Work out the finished part from the listing and answer in its coordinate system (mm). A direction names the side the tool comes from. Give positions to 0.01 mm unless a question says otherwise; leave off trailing zeros. Order: outer loops, then holes, each group sorted by start corner. A loop starts at its lowest first (then second) coordinate and runs counter-clockwise, first axis right, second up. Notation, with made-up numbers: M 3.5,-0.5 L 7.5,-0.5 A10 cw 7.5,4.5 Z; hole C 24.25,-4.75 d8. An arc over 180 degrees is marked long. One line per item, written item: value.
Autodesk Inventor part; units mm, degrees
ref_plane "YZ Plane" through (0, 0, 0) normal (1, 0, 0) x (0, 1, 0)
ref_plane "XZ Plane" through (0, 0, 0) normal (0, 1, 0) x (-1, 0, 0)
ref_plane "XY Plane" through (0, 0, 0) normal (0, 0, 1) x (1, 0, 0)
sketch "스케치1" plane through (0, 0, 0) normal (0, 1, 0) x (-1, 0, 0)
  line L0 (22.5, -14) -> (-22.5, -14)
  line L1 (-22.5, -14) -> (-22.5, 14)
  line L2 (-22.5, 14) -> (22.5, 14)
  line L3 (22.5, 14) -> (22.5, -14)
  point P0 (0, 0)
  dimension "d0" = 28
  dimension "d1" = 45
  dimension "d2" = 14
  dimension "d3" = 22.5
extrude "돌출1" add sketch "스케치1" along normal blind 5
sketch "스케치2" plane through (0, 5, 0) normal (0, 1, 0) x (1, 0, 0)
  circle A0 centre (18.5, 0) radius 5
  line L0 (18.5, 5) -> (22.5, 5)
  line L1 (22.5, 5) -> (22.5, -5)
  line L2 (22.5, -5) -> (18.5, -5)
  line L3 (18.5, -5) -> (18.5, 5)
  line L4 (22.5, -14) -> (22.5, 14)
  point P0 (0, 0)
  dimension "d6" = 10
  dimension "d7" = 0
  dimension "d8" = 10
  dimension "d9" = 5
  dimension "d10" = 4
  dimension "d11" = 0
extrude "돌출2" cut sketch "스케치2" against normal blind 100
sketch "스케치3" plane through (0, 5, 0) normal (0, 1, 0) x (1, 0, 0)
  circle A0 centre (19.5, 11) radius 1.25
  line L0 (22.5, 5) -> (22.5, 14)
  line L1 (22.5, 14) -> (-22.5, 14)
  line L2 (0, 0) -> (4.9885, 0)
  circle A1 centre (19.5, -11) radius 1.25
  circle A2 centre (8.5, 0) radius 1.25
  line L3 (-22.5, -14) -> (22.5, -14)
  circle A3 centre (11.722, -7.778) radius 1.25
  line L4 (22.5, -14) -> (22.5, -5)
  circle A4 centre (11.722, 7.778) radius 1.25
  dimension "d14" = 2.5
  dimension "d15" = 3
  dimension "d16" = 3
  dimension "d17" = 14
  dimension "d18" = 2.5
  dimension "d19" = 14
  dimension "d20" = 10.778
  dimension "d21" = 6.222
  dimension "d22" = 2.5
extrude "돌출3" cut sketch "스케치3" against normal blind 5
fillet "모깎기1" radius 2 4 edges at (22.5, 2.5, -14) (22.5, 2.5, 14) (22.5, 2.5, -5) (22.5, 2.5, 5)
sketch "스케치4" plane through (0, 0, 0) normal (0, -1, 0) x (1, 0, 0)
  line L0 (-22.5, -14) -> (20.5, -14)
  line L1 (20.5, 14) -> (-22.5, 14)
  line L2 (-22.5, -14) -> (-17.5, -14)
  line L3 (-17.5, -14) -> (-17.5, 14)
  line L4 (-17.5, 14) -> (-22.5, 14)
  line L5 (-22.5, 14) -> (-22.5, -14)
  point P0 (0, 0)
  dimension "d26" = 5
extrude "돌출4" add sketch "스케치4" along normal blind 52
fillet "모깎기2" radius 2 1 edges at (-22.5, 5, 0)
sketch "스케치5" plane through (-17.5, 0, 14) normal (1, 0, 0) x (0, 0, -1)
  point P0 (14, 0)
sketch "스케치6" plane through (-17.5, 0, 14) normal (1, 0, 0) x (0, 0, -1)
  line L0 (28, 0) -> (28, -52)
  line L1 (0, 0) -> (0, -52)
  line L2 (28, -52) -> (0, -52)
  line L3 (0, -52) -> (0, -47)
  line L4 (0, -47) -> (28, -47)
  line L5 (28, -47) -> (28, -52)
  point P0 (14, 0)
  dimension "d30" = 5
extrude "돌출5" add sketch "스케치6" along normal blind 40
sketch "스케치7" plane through (0, 0, 0) normal (0, -1, 0) x (1, 0, 0)
  circle A0 centre (19.5, -11) radius 1.25
  circle A1 centre (19.5, -11) radius 1.25
  circle A2 centre (11.722, -7.778) radius 1.25
  circle A3 centre (11.722, -7.778) radius 1.25
  circle A4 centre (8.5, 0) radius 1.25
  circle A5 centre (8.5, 0) radius 1.25
  circle A6 centre (11.722, 7.778) radius 1.25
  circle A7 centre (11.722, 7.778) radius 1.25
  circle A8 centre (19.5, 11) radius 1.25
  circle A9 centre (19.5, 11) radius 1.25
  arc A10 (18.5, 5) -> (18.5, -5) centre (18.5, 0) ccw
  circle A11 centre (18.5, 0) radius 5
  line L0 (18.5, -5) -> (29.1098, -5)
  line L1 (29.1098, -5) -> (29.1098, 5)
  line L2 (29.1098, 5) -> (18.5, 5)
  line L3 (18.5, 5) -> (18.5, -5)
  point P0 (0, 0)
extrude "돌출6" cut sketch "스케치7" along normal blind 200
fillet "모깎기4" radius 2 2 edges at (22.5, -49.5, 14) (22.5, -49.5, -14)
fillet "모깎기5" radius 2 1 edges at (-22.5, -52, 0)
sketch "스케치10" plane through (20.5, 0, 14) normal (0, 0, 1) x (1, 0, 0)
  circle A0 centre (-41, -12.5) radius 1.5
  circle A1 centre (-41, -34.5) radius 1.5
  line L0 (-32.0554, -23.5) -> (-2.5003, -23.5)
  line L1 (-43, 3) -> (-43, -50)
  point P0 (-20.5, 0)
  dimension "d54" = 3
  dimension "d55" = 3
  dimension "d56" = 22
  dimension "d57" = 23.5
  dimension "d58" = 11
  dimension "d59" = 2
  dimension "d60" = 2
extrude "돌출9" cut sketch "스케치10" against normal blind 80
sketch "스케치11" plane through (-17.5, 0, 14) normal (1, 0, 0) x (0, 0, -1)
  line L0 (5, -42) -> (23, -42)
  line L1 (23, -42) -> (23, -5)
  line L2 (23, -5) -> (5, -5)
  line L3 (5, -5) -> (5, -42)
  line L4 (0, 0) -> (0, -47)
  line L5 (28, 0) -> (28, -47)
  line L6 (19, 0) -> (9, 0)
  line L7 (9, -47) -> (19, -47)
  line L8 (11, -42) -> (17, -42)
  line L9 (17, -42) -> (17, -5)
  line L10 (17, -5) -> (11, -5)
  line L11 (11, -5) -> (11, -42)
  point P0 (14, 0)
  dimension "d63" = 5
  dimension "d64" = 5
  dimension "d65" = 5
  dimension "d66" = 5
  dimension "d67" = 6
  dimension "d68" = 6
extrude "돌출10" cut sketch "스케치11" against normal blind 80 contours L3 L2 L11 L0 | L9 L2 L1 L0
sketch "스케치12" plane through (-17.5, -42, 3) normal (0, 0, 1) x (1, 0, 0)
  circle A0 centre (-3, 7.5) radius 1.5
  circle A1 centre (-3, 7.5) radius 1.5
  circle A2 centre (-3, 29.5) radius 1.5
  circle A3 centre (-3, 29.5) radius 1.5
  point P0 (17.5, 42)
extrude "돌출11" add sketch "스케치12" against normal blind 6
properties part number "elbow_gear"
(1) Section D-D, the plane z = 0 is taken. Give the vertices of the cut face in (x, y), then the cut area to 3 significant figures.
Findings:
outline: M -22.5,-50 A2 ccw -20.5,-52 L 7.25,-52 L 7.25,-47 L -17.5,-47 L -17.5,0 L 7.25,0 L 7.25,5 L -20.5,5 A2 ccw -22.5,3 Z; M 9.75,-52 L 13.5,-52 L 13.5,-47 L 9.75,-47 Z; M 9.75,0 L 13.5,0 L 13.5,5 L 9.75,5 Z
area: 568 mm^2
(2) Find the intervals of material crossed by probe 1 along Z at (x, y) = (19.5, -50.55); probe 2 along Z at (x, y) = (-19, -18.5); probe 3 along Y at (x, z) = (-10, -10), in increasing order. Write a range as from..to.
Findings:
probe 1: z = -14..-12.25, -9.75..-5, 5..9.75, 12.25..14
probe 2: z = -14..-9, -3..3, 9..14
probe 3: y = -52..-47, 0..5
(3) Determine the mould class of faces 1 (the flat face through (22.5, 2, 9)), 2 (the cylindrical face through (20.69, -49.46, 10.62)), 3 (the flat face through (-19, -23, 14)), 4 (the cylindrical face through (12.299, 2.535, 8.887)) for opening direction Z: pulls with the +Z half, pulls with the -Z half, needs draft (parallel to the pull), parting line crosses it, or undercut.
Findings:
face 1: needs draft
face 2: undercut
face 3: pulls with the +Z half
face 4: undercut
(4) Section C-C, the plane y = -23.5 is taken. Give the vertices of the cut face in (x, z).
Findings:
outline: M -22.5,-14 L -17.5,-14 L -17.5,-9 L -22.5,-9 Z; M -22.5,-3 L -17.5,-3 L -17.5,3 L -22.5,3 Z; M -22.5,9 L -17.5,9 L -17.5,14 L -22.5,14 Z
(5) Section A-A, the plane z = 11 is taken. Give the vertices of the cut face in (x, y), then the cut area to 3 significant figures.
Findings:
outline: M -22.5,-50 A2 ccw -20.5,-52 L 18.25,-52 L 18.25,-47 L -17.5,-47 L -17.5,0 L 18.25,0 L 18.25,5 L -20.5,5 A2 ccw -22.5,3 Z; M 20.75,-52 L 22.5,-52 L 22.5,-47 L 20.75,-47 Z; M 20.75,0 L 22.5,0 L 22.5,5 L 20.75,5 Z; hole C -20.5,-34.5 d3; hole C -20.5,-12.5 d3
area: 644 mm^2
(6) Section B-B, the plane x = -15.5 is taken. Give the vertices of the cut face in (y, z).
Findings:
outline: M -52,-14 L -47,-14 L -47,14 L -52,14 Z; M 0,-14 L 5,-14 L 5,14 L 0,14 Z
(7) Which of the six approach directions +Z, -Z, +X, -X, +Y, -Y give full straight-line access (tool end or side, diameter ignored) to faces 5 (the cylindrical face through (-21.7, -35.4, -11.5)), 6 (the cylindrical face through (-22, -12.43, 11.54)), 7 (the flat face through (-20, -42, -6)), 8 (the flat face through (21, -49, 5)), 9 (the cylindrical face through (21.9, 2.46, 5.57))?
Findings:
face 5: -Z
face 6: +Z
face 7: +X, -X
face 8: +X, +Y, -Y
face 9: +X, +Y
(8) Given P1, Ø2.5, axis at x = -20.5, y = -34.5, coming from the -Z side; P2, Ø1.8, axis at x = -20.5, y = -12.5, coming from the +Z side, each flat-ended and moving along its own axis, determine where each tip first touches the part or whether it passes through.
Findings:
P1: stops at z = -3
P2: stops at z = 3
